Design review of the part built by this model. Coordinates are the model's own, in mm. A direction names the side the tool comes from. Round coordinates to 2 decimals unless told otherwise and drop trailing zeros. Loops run counter-clockwise (first coordinate to the right, second up) from the corner with the lowest first, then second, coordinate; pieces in that order, holes last. Notation, with made-up numbers: M -33.75,-1.5 L 19.25,-1.5 A24 ccw 19.25,28.5 Z; hole C -1,89 d5. An arc over 180 degrees is marked long. Use a Markdown table: item, result.
from build123d import *

# Parameters (mm, degrees)
BOSS_EXTRUDE1_DEPTH = 1
SKETCH2_W           = 50
SKETCH2_H           = 11.4
BOSS_EXTRUDE2_DEPTH = 4.4
SKETCH3_R           = 2.25
CUT_EXTRUDE1_DEPTH  = 4.4
SKETCH4_W           = 50.6
SKETCH4_H           = 5.5
BOSS_EXTRUDE3_DEPTH = 6.4
SKETCH5_W           = 50.6
SKETCH5_H           = 4.5
BOSS_EXTRUDE4_DEPTH = 1.8
SKETCH6_W           = 50.6
SKETCH6_H           = 5.5
BOSS_EXTRUDE5_DEPTH = 2


with BuildPart() as part:
    # Sketch1 → Boss-Extrude1 (new body)
    with BuildSketch(Plane(origin=(0, 0, 0), x_dir=(0, 1, 0), z_dir=(0, 0, 1))):
        Polygon((-25, 25.3), (19, 25.3), (25, 25.3), (25, -25.3), (-25, -25.3), align=None)
    extrude(amount=BOSS_EXTRUDE1_DEPTH)

    # Sketch2 → Boss-Extrude2 (add)
    with BuildSketch(Plane.YZ.offset(25.3)):
        with Locations((0, -4.7)):
            Rectangle(SKETCH2_W, SKETCH2_H)
    extrude(amount=BOSS_EXTRUDE2_DEPTH)

    # Sketch3 → Cut-Extrude1 (cut)
    with BuildSketch(Plane.YZ.offset(29.7)):
        with Locations(Location((-20, -3.787139035, 0), (0, 0, 270))):
            Circle(SKETCH3_R)
        with Locations(Location((20, -3.787139035, 0), (0, 0, 270))):
            Circle(SKETCH3_R)
    extrude(amount=-CUT_EXTRUDE1_DEPTH, mode=Mode.SUBTRACT)

    # Sketch4 → Boss-Extrude3 (add)
    with BuildSketch(Plane(origin=(0, 0, 0), x_dir=(1, 0, 0), z_dir=(0, 0, -1))):
        with Locations((0, -22.25)):
            Rectangle(SKETCH4_W, SKETCH4_H)
        with Locations((0, 22.25)):
            Rectangle(SKETCH4_W, SKETCH4_H)
    extrude(amount=BOSS_EXTRUDE3_DEPTH)

    # Sketch5 → Boss-Extrude4 (add)
    with BuildSketch(Plane(origin=(0, 0, -6.4), x_dir=(1, 0, 0), z_dir=(0, 0, -1))):
        with Locations((0, 22.75)):
            Rectangle(SKETCH5_W, SKETCH5_H)
        with Locations((0, -22.75)):
            Rectangle(SKETCH5_W, SKETCH5_H)
    extrude(amount=BOSS_EXTRUDE4_DEPTH)

    # Sketch6 → Boss-Extrude5 (add)
    with BuildSketch(Plane(origin=(0, 0, -8.2), x_dir=(1, 0, 0), z_dir=(0, 0, -1))):
        with Locations((0, -22.25)):
            Rectangle(SKETCH6_W, SKETCH6_H)
        with Locations((0, 22.25)):
            Rectangle(SKETCH6_W, SKETCH6_H)
    extrude(amount=BOSS_EXTRUDE5_DEPTH)


solid = part.part
1. The part is to be moulded in two halves that separate along Y. For faces 1 (the face through (2, -25, -5)), 2 (the face through (0, -19.5, -3)), 3 (the face through (29.7, 0, -5)), say which applies: pulls with the +Y half, pulls with the -Y half, needs draft (parallel to the pull), parting line crosses it, or undercut.
Check values:
| item | result |
|---|---|
| face 1 | pulls with the -Y half |
| face 2 | undercut |
| face 3 | needs draft |
2. Take a section at A-A on y = 18.5. Give the boundary of the cut face in (x, z).
Check values:
| item | result |
|---|---|
| outline | M -25.3,0 L 25.3,0 L 25.3,-2.11 L 29.7,-2.11 L 29.7,1 L -25.3,1 Z; M 25.3,-10.4 L 29.7,-10.4 L 29.7,-5.46 L 25.3,-5.46 Z |
3. Take a section at D-D on y = 4. Give the boundary of the cut face in (x, z).
Check values:
| item | result |
|---|---|
| outline | M -25.3,0 L 25.3,0 L 25.3,-10.4 L 29.7,-10.4 L 29.7,1 L -25.3,1 Z |
4. Take a section at C-C on x = 13.5. Give the boundary of the cut face in (y, z), and give its area (3 significant figures).
Check values:
| item | result |
|---|---|
| outline | M -25,-10.2 L -19.5,-10.2 L -19.5,-8.2 L -20.5,-8.2 L -20.5,-6.4 L -19.5,-6.4 L -19.5,0 L 19.5,0 L 19.5,-6.4 L 20.5,-6.4 L 20.5,-8.2 L 19.5,-8.2 L 19.5,-10.2 L 25,-10.2 L 25,1 L -25,1 Z |
| area | 159 mm² |
5. Take a section at B-B on z = -9. Give the boundary of the cut face in (x, y), and give its area (3 significant figures).
Check values:
| item | result |
|---|---|
| outline | M -25.3,-25 L 29.7,-25 L 29.7,25 L -25.3,25 L -25.3,19.5 L 25.3,19.5 L 25.3,-19.5 L -25.3,-19.5 Z |
| area | 777 mm² |
6. Wall thickness on line 1 along Y through (x, z) = (10, -8.5); line 2 along Z through (x, y) = (26.4, -20); line 3 along Y through (x, z) = (-6.5, -6.75): over which ranges is each line inside the solid? List them lowest first. Write a range as from..to.
Check values:
| item | result |
|---|---|
| line 1 | y = -25..-19.5, 19.5..25 |
| line 2 | z = -10.4..-6.04, -1.54..1 |
| line 3 | y = -25..-20.5, 20.5..25 |
7. Insertion check: pin 1 (1.1 mm diameter, centred on x = 4, y = -20, fed in from -Z); pin 2 (5 mm diameter, centred on y = 10.5, z = -6, fed in from -X); pin 3 (3 mm diameter, centred on y = 20.5, z = -4, fed in from +X). Each pin has a flat end and moves straight along its axis. Give the tip position at first contact, or say it passes through.
Check values:
| item | result |
|---|---|
| pin 1 | stops at z = -10.2 |
| pin 2 | stops at x = 25.3 |
| pin 3 | stops at x = 25.3 |
8. Machinability: for faces 4 (the face through (0, -20.5, -7)), 5 (the face through (0, -19.5, -9)), 6 (the face through (25.3, 21, -4)), 7 (the face through (0, -22, -10.2)), which of the approach directions +Z, -Z, +X, -X, +Y, -Y give a long, thin tool a straight path to every point of the face, cutting with its end or side? Answer none if there is none.
Check values:
| item | result |
|---|---|
| face 4 | -X |
| face 5 | -Z, -X |
| face 6 | +X |
| face 7 | -Z, -X, +Y, -Y |
